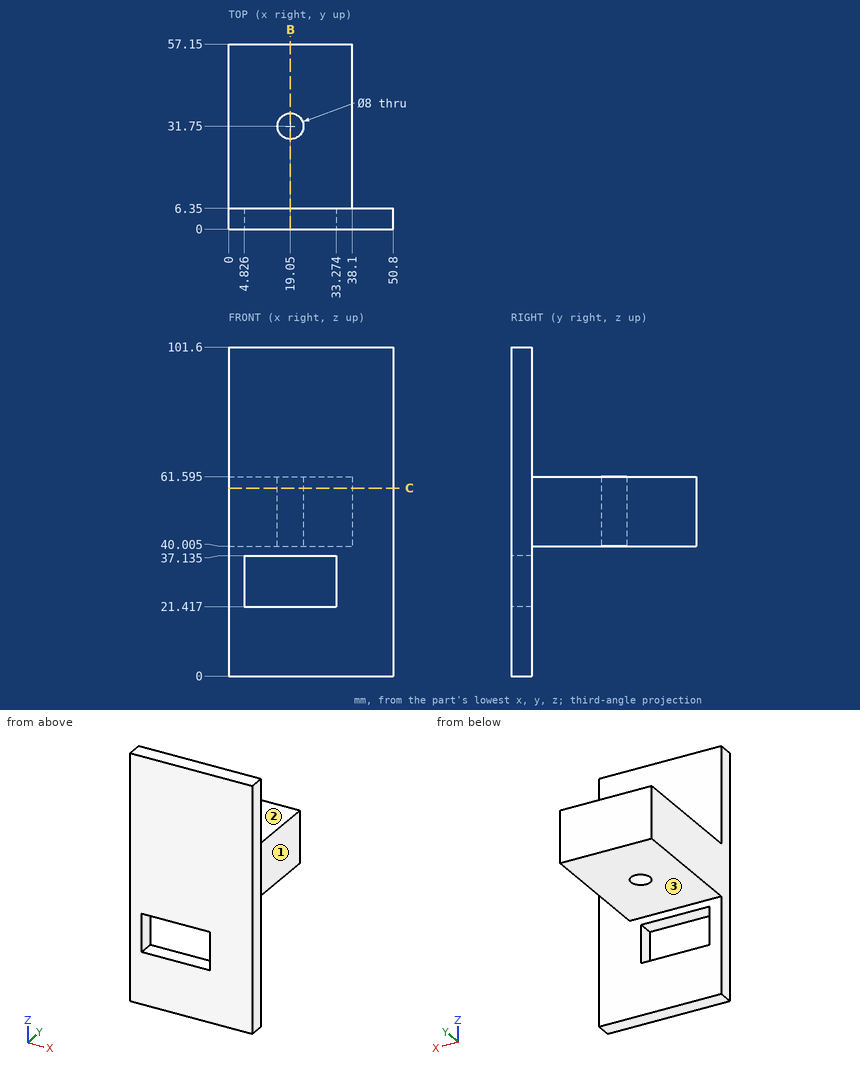
Could you check a few things on this drawing? It's one solid part, dimensions in mm from its lowest x, y, z. A direction names the side the tool comes from. Coordinates: 2 decimals unless noted, no trailing zeros. Write each loop counter-clockwise with the first axis right and the second up, starting at its lowest first coordinate (ties: lowest second). Pieces come first, ordered by that corner, then holes. Notation, with made-up numbers: (0, 51) - (9, 51) arc R26 ccw to (9, 78) - close; hole circle Ø11 at (68, 23.5). An arc over 180 degrees is marked (long way). Write item = value, one per line.
1) For the marked faces 1, 2 and 3, which set-ups out of +Z, -Z, +X, -X, +Y, -Y let a thin tool reach every point of the face, with its end or its side?
Result set:
face_1 = +Z, -Z, +X, +Y
face_2 = +Z, +X, -X, +Y
face_3 = -Z, +X, -X, +Y
2) Will these pins go through, and if not, where does the flat tip stop? pin 1 Ø4 at (x, y) = (37, 19) entering from +Z (3 decimals); pin 2 Ø1 at (y, z) = (7.5, 44.5) entering from +X.
Result set:
pin_1 = 61.595
pin_2 = 38.1
3) Suppose I cut it at B-B on x = 19.05. State how many separate pieces and enclosed holes the cut face has, plus the area to 3 significant figures.
Result set:
separate_pieces = 3
enclosed_holes = 0
area = 1,470 mm2
4) Please list where these lines run through material, in increasing order: line 1 (Y direction, x = 19.05, z = 46); line 2 (X direction, y = 3, z = 24.5); line 3 (Y direction, x = 39, z = 90). Write a range as [from, to].
Result set:
line_1 = [0, 27.75], [35.75, 57.15]
line_2 = [0, 4.83], [33.27, 50.8]
line_3 = [0, 6.35]
5) Suppose I cut it at C-C on z = 58. Please give me the cut outline in (x, y).
Result set:
outline = (0, 0) - (50.8, 0) - (50.8, 6.35) - (38.1, 6.35) - (38.1, 57.15) - (0, 57.15) - close; hole circle Ø8 at (19.05, 31.75)
